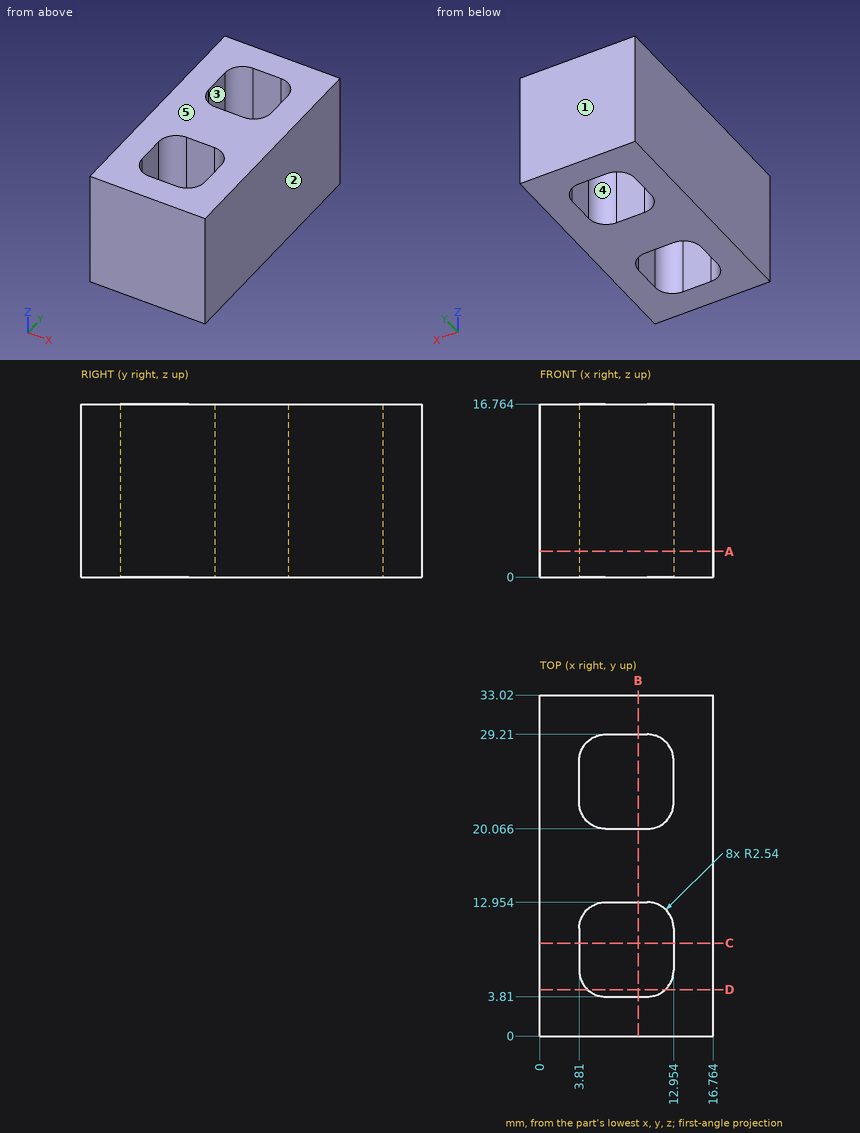
Print and shaded views of the part. All mm, measured from the part's lowest x, y and z. A direction names the side the tool comes from. Coordinates: 2 decimals unless noted, no trailing zeros. Order: outer loops, then holes, each group sorted by start corner. A loop starts at its lowest first (then second) coordinate and runs counter-clockwise, first axis right, second up.
Item 1: Drop a flat-ended pin along its axis: pin 1 Ø10 at (x, z) = (4, 13) entering from -Y. Give the stop position or say it passes through.
Filled in:
pin 1: stops at y = 0
Item 2: Drill centre lines: L1, parallel to Y at x = 9.25, z = 13; L2, parallel to X at y = 8.5, z = 2.75; L3, parallel to Y at x = 5.5, z = 5.75. Where is each one in solid material? Low to high.
Filled in:
L1: y = 0 to 3.81, 12.95 to 20.07, 29.21 to 33.02
L2: x = 0 to 3.81, 12.95 to 16.76
L3: y = 0 to 3.96, 12.81 to 20.21, 29.06 to 33.02
Item 3: Saw through at C-C on y = 9. List the corners of the cut face in (x, z), then the cut area to 3 significant figures.
Filled in:
outline: (0, 0) - (3.81, 0) - (3.81, 16.76) - (0, 16.76) - close; (12.95, 0) - (16.76, 0) - (16.76, 16.76) - (12.95, 16.76) - close
area: 128 mm2
Item 4: Mould opens along Y. For the marked faces 1, 2 and 3 say: released by +Y, released by -Y, zero draft, split by the parting line, or undercut.
Filled in:
face 1: released by +Y
face 2: zero draft
face 3: undercut
Item 5: Saw through at D-D on y = 4.5. List the corners of the cut face in (x, z).
Filled in:
outline: (0, 0) - (4.61, 0) - (4.61, 16.76) - (0, 16.76) - close; (12.15, 0) - (16.76, 0) - (16.76, 16.76) - (12.15, 16.76) - close
Item 6: Saw through at A-A on z = 2.5. List the corners of the cut face in (x, y).
Filled in:
outline: (0, 0) - (16.76, 0) - (16.76, 33.02) - (0, 33.02) - close; hole (3.81, 6.35) arc R2.54 ccw to (6.35, 3.81) - (10.41, 3.81) arc R2.54 ccw to (12.95, 6.35) - (12.95, 10.41) arc R2.54 ccw to (10.41, 12.95) - (6.35, 12.95) arc R2.54 ccw to (3.81, 10.41) - close; hole (3.81, 22.61) arc R2.54 ccw to (6.35, 20.07) - (10.41, 20.07) arc R2.54 ccw to (12.95, 22.61) - (12.95, 26.67) arc R2.54 ccw to (10.41, 29.21) - (6.35, 29.21) arc R2.54 ccw to (3.81, 26.67) - close
Item 7: Saw through at B-B on x = 9.5. List the corners of the cut face in (y, z), then the cut area to 3 significant figures.
Filled in:
outline: (0, 0) - (3.81, 0) - (3.81, 16.76) - (0, 16.76) - close; (12.95, 0) - (20.07, 0) - (20.07, 16.76) - (12.95, 16.76) - close; (29.21, 0) - (33.02, 0) - (33.02, 16.76) - (29.21, 16.76) - close
area: 247 mm2
Item 8: Tool access for the marked faces 4 and 5: list every direction of +Z, -Z, +X, -X, +Y, -Y with a clear straight run to the whole face (end or side of a thin tool).
Filled in:
face 4: +Z, -Z
face 5: +Z, +X, -X, +Y, -Y
